```python
from build123d import *

# Parameters (mm, degrees)
SKETCH1_W           = 121
SKETCH1_H           = 55
BOSS_EXTRUDE1_DEPTH = 4
SKETCH1_3_W         = 12.5
SKETCH1_3_H         = 3.4


with BuildPart() as part:
    # Sketch1 → Boss-Extrude1 (new, symmetric)
    with BuildSketch(Plane(origin=(0, 0, 0), x_dir=(1, 0, 0), z_dir=(0, 1, 0))):
        Rectangle(SKETCH1_W, SKETCH1_H)
    extrude(amount=BOSS_EXTRUDE1_DEPTH, both=True)

    # Sketch1_3 → Revolve1 (revolve)
    with BuildSketch(Plane(origin=(0, 0, 0), x_dir=(1, 0, 0), z_dir=(0, 1, 0)), mode=Mode.PRIVATE) as revolve1_sk:
        with Locations((-66.75, 20.8)):
            Rectangle(SKETCH1_3_W, SKETCH1_3_H)
    revolve1 = revolve(revolve1_sk.sketch.rotate(Axis((-73, 0, -19.1), (1, 0, 0)), 180), axis=Axis((-73, 0, -19.1), (1, 0, 0)))

    # Mirror1: Revolve1 across plane
    add(revolve1.mirror(Plane(origin=(0, 0, 0), x_dir=(0, 0, 1), z_dir=(1, 0, 0))))


solid = part.part
```
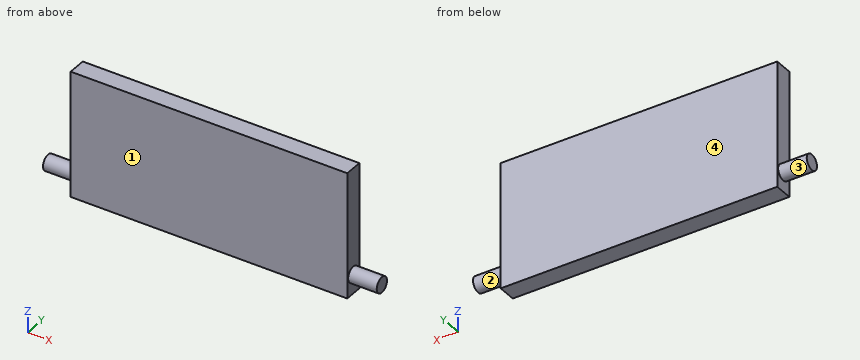
Here's how the part is built. I have some questions about the finished solid (model axes, mm). Face numbers are marked on the shaded views. A direction names the side the tool comes from. Round coordinates to 2 decimals unless told otherwise and drop trailing zeros. Order: outer loops, then holes, each group sorted by start corner. A loop starts at its lowest first (then second) coordinate and runs counter-clockwise, first axis right, second up. Notation, with made-up numbers: M 47.25,15 L 56.25,15 A28 cw 56.25,51 Z; hole C 56,35 d4. An arc over 180 degrees is marked long. Use CSV: the item, a comma, the result in double quotes.
1) I want a section at C-C (x = 64). List the corners of the cut face in (y, z) for me, then the cut area to 3 significant figures.
Taken from the geometry:
outline,"C 0,-19.1 d6.8"
area,"36.3 mm^2"
2) I want a section at D-D (z = 0.5). List the corners of the cut face in (x, y) for me.
Taken from the geometry:
outline,"M -60.5,-4 L 60.5,-4 L 60.5,4 L -60.5,4 Z"
3) I want a section at B-B (z = -19.1). List the corners of the cut face in (x, y) for me, then the cut area to 3 significant figures.
Taken from the geometry:
outline,"M -73,-3.4 L -60.5,-3.4 L -60.5,-4 L 60.5,-4 L 60.5,-3.4 L 73,-3.4 L 73,3.4 L 60.5,3.4 L 60.5,4 L -60.5,4 L -60.5,3.4 L -73,3.4 Z"
area,"1,140 mm^2"
4) I want a section at A-A (y = 0). List the corners of the cut face in (x, z) for me.
Taken from the geometry:
outline,"M -73,-22.5 L -60.5,-22.5 L -60.5,-27.5 L 60.5,-27.5 L 60.5,-22.5 L 73,-22.5 L 73,-15.7 L 60.5,-15.7 L 60.5,27.5 L -60.5,27.5 L -60.5,-15.7 L -73,-15.7 Z"
5) I need wall thicknesses on line 1 along X through (y, z) = (0.75, 10); line 2 along Z through (x, y) = (67.5, 0.25). Which ranges of each line are inside material? Lowest first, please. Write a range as [from, to].
Taken from the geometry:
line 1,"[-60.5, 60.5]"
line 2,"[-22.49, -15.71]"
6) I'm going to push flat-ended pins straight in: P1, Ø4, axis at y = 2.5, z = 6.5, coming from the -X side; P2, Ø1.5, axis at y = -2.5, z = 0, coming from the +X side. Where does each tip first touch, or does it pass through?
Taken from the geometry:
P1,"x = -60.5"
P2,"x = 60.5"
7) On a 3-axis mill with a long thin cutter (end or side, diameter ignored), from which of +Z, -Z, +X, -X, +Y, -Y can I reach the whole of each face in a straight line? I mean the marked faces 1 and 2. Say none if no direction works.
Taken from the geometry:
face 1,"+Z, -Z, +X, -X, -Y"
face 2,"+X"
8) If we mould it in two halves opening along Z, with no side actions, what happens to the marked faces 3 and 4? For each: pulls with the +Z half, pulls with the -Z half, needs draft (parallel to the pull), parting line crosses it, or undercut.
Taken from the geometry:
face 3,"parting line crosses it"
face 4,"needs draft"
